```python
from build123d import *

# Parameters (mm, degrees)
F0_R     = 32.895129
F1_DEPTH = 70
F2_SIZE  = 2
F3_SIZE  = 2
F4_T     = -2.5


with BuildPart() as f1:
    # F0 (on Top) → F1 (new body)
    with BuildSketch(Plane.XY):
        with Locations((-31.053945, 27.464956)):
            Circle(F0_R)
    extrude(amount=F1_DEPTH)

    # F2
    f2_edges = [f1.edges().sort_by_distance(p)[0] for p in [
        (-63.949075, 27.464956, 70),
    ]]
    chamfer(f2_edges, length=F2_SIZE)

    # F3
    f3_edges = [f1.edges().sort_by_distance(p)[0] for p in [
        (-63.949075, 27.464956, 0),
    ]]
    chamfer(f3_edges, length=F3_SIZE)

    # F4
    f4_openings = [f1.faces().sort_by_distance(p)[0] for p in [
        (-31.053945, 27.464956, 70),
    ]]
    offset(amount=F4_T, openings=f4_openings)


solid = f1.part
```
Source: CAD feature listing. Evaluate the final solid. Frame: model axes, mm. A direction names the side the tool comes from. Round coordinates to 2 decimals unless told otherwise and drop trailing zeros. Loops run counter-clockwise (first coordinate to the right, second up) from the corner with the lowest first, then second, coordinate; pieces in that order, holes last. Notation, with made-up numbers: M 2.25,19.25 L 29.25,19.25 A31 ccw 29.25,56.25 Z; hole C 52,85 d3. An arc over 180 degrees is marked long. Put each result on its own line as item: value.
(1) Access query for faces 1 (the face through (-13.37, 55.202, 34.538)), 2 (the face through (-31, 28, 2.5)). Directions: +Z, -Z, +X, -X, +Y, -Y. A direction counts if a zero-diameter tool reaches every point of the face in a straight line with its end or side. Return the directions, or none.
Solutions:
face 1: +Z, -Z
face 2: none
(2) Ray query, line 1 (Z direction, x = -2, y = 31.5); line 2 (Z direction, x = -14.5, y = 13); line 3 (X direction, y = 36, z = 20). Return the intervals inside material, ascending. Write a range as [from, to].
Solutions:
line 1: [0, 2.5], [68.03, 70]
line 2: [0, 2.5]
line 3: [-62.82, -60.23], [-1.88, 0.71]
(3) Section A-A, the plane z = 19.5. Return loops of the section in (x, y), and give its area (3 significant figures).
Solutions:
outline: C -31.05,27.46 d65.79; hole C -31.05,27.46 d60.79
area: 497 mm²
(4) Pull-direction query (Z, two-part tool) for faces 3 (the face through (-34.63, 54.74, 69.85)), 4 (the face through (-53.456, 48.007, 34.552)), 5 (the face through (-31, 28, 0)), 6 (the face through (-50, 7, 70)); classes: released by +Z, released by -Z, zero draft, split by the parting line, or undercut.
Solutions:
face 3: undercut
face 4: undercut
face 5: released by -Z
face 6: released by +Z
(5) First-contact query: pin 1 (8 mm diameter, centred on x = -46.5, z = 13, fed in from +Y); pin 2 (1 mm diameter, centred on x = -10, y = 35.5, fed in from -Z); pin 3 (2 mm diameter, centred on y = 29.5, z = 30.5, fed in from +X); pin 4 (1 mm diameter, centred on y = 23, z = 46, fed in from -X). Flat tips, straight axial feed; report the tip coordinate or a pass-through.
Solutions:
pin 1: y = 58.3
pin 2: z = 0
pin 3: x = 1.82
pin 4: x = -63.71
